```python
from build123d import *

# Parameters (mm, degrees)
EXTRUDE_1_DEPTH     = 3
SKETCH_5_R          = 1.65
CUT_EXTRUDE_1_DEPTH = 8


with BuildPart() as part:
    # Эскиз1 → Бобышка-Вытянуть1 (new body)
    with BuildSketch(Plane.XY):
        Polygon((0, 0), (0, 200), (50, 150), (50, 50), align=None)
    extrude(amount=EXTRUDE_1_DEPTH)

    # Эскиз5 → Вырез-Вытянуть1 (cut)
    with BuildSketch(Plane(origin=(-305.961161651, -184.204468703, -1.5), x_dir=(-0.9998892265297747, 0.01488404077153568, 0), z_dir=(0, 0, -1))):
        with BuildLine():
            ThreePointArc((-309.659295343, 358.877763083), (-310.142569154, 360.044489272), (-311.309295343, 360.527763083))
            Line((-311.309295343, 360.527763083), (-311.309295343, 357.227763083))
            ThreePointArc((-311.309295343, 357.227763083), (-310.142569154, 357.711036894), (-309.659295343, 358.877763083))
        make_face()
        with BuildLine():
            Line((-311.309295343, 357.227763083), (-311.309295343, 360.527763083))
            ThreePointArc((-311.309295343, 360.527763083), (-312.959295343, 358.877763083), (-311.309295343, 357.227763083))
        make_face()
        with Locations(Location((-311.309295343, 218.877763083, 0), (0, 0, 179.147175791))):
            Circle(SKETCH_5_R)
    extrude(amount=-CUT_EXTRUDE_1_DEPTH, mode=Mode.SUBTRACT)


solid = part.part
```
Here's how the part is built. I have some questions about the finished solid (model axes, mm). Coordinates: 2 decimals unless noted, no trailing zeros. Order: outer loops, then holes, each group sorted by start corner. A loop starts at its lowest first (then second) coordinate and runs counter-clockwise, first axis right, second up. Notation, with made-up numbers: M 59,78.5 L 97,78.5 A19 ccw 97,90.5 Z; hole C 17,77.25 d8. An arc over 180 degrees is marked long. Answer as a JSON object with one key per item and string values. Group by question number.
(1) Suppose I cut it at C-C, the plane x = 28. Please give me the cut outline in (y, z).
(2) I need wall thicknesses on probe 1 along Y at (x, z) = (10, 0.35); probe 2 along Y at (x, z) = (11.5, 2.75); probe 3 along X at (y, z) = (30, 1.05). Which ranges of each line are inside material? Lowest first, please.
(3) If we mould it in two halves opening along Y, with no side actions, what happens to faces 1 (the face through (25, 175, 1)), 2 (the face through (9.458, 28.624, 1.479)), 3 (the face through (20, 101, 3)), 4 (the face through (25, 25, 1))? For each: released by +Y, released by -Y, zero draft, split by the parting line, or undercut.
(4) For pin 1 (3 mm diameter, centred on x = 43, y = 39, fed in from +Z); pin 2 (1 mm diameter, centred on x = 12.5, y = 120, fed in from -Z); pin 3 (1 mm diameter, centred on x = 11, z = 2.5, fed in from +Y); pin 4 (1.5 mm diameter, centred on x = 18.5, z = 0.5, fed in from +Y), each with a flat end and sliding along its axis, tell me the tip position at first contact or that it passes through.
(5) Suppose I cut it at B-B, the plane y = 153. Please give me the cut outline in (x, z).
(6) Suppose I cut it at A-A, the plane z = 2.1. Please give me the cut outline in (x, y), then the cut area to 3 significant figures.
Values found:
{
 "1": {"outline": "M 28,0 L 172,0 L 172,3 L 28,3 Z"},
 "2": {"probe 1": "y = 10 to 29.19, 30.84 to 168.49, 171.51 to 190", "probe 2": "y = 11.5 to 168.58, 171.42 to 188.5", "probe 3": "x = 0 to 6.92, 10.22 to 30"},
 "3": {"face 1": "released by +Y", "face 2": "undercut", "face 3": "zero draft", "face 4": "released by -Y"},
 "4": {"pin 1": "passes through", "pin 2": "stops at z = 0", "pin 3": "stops at y = 189.5", "pin 4": "stops at y = 182.25"},
 "5": {"outline": "M 0,0 L 47,0 L 47,3 L 0,3 Z"},
 "6": {"outline": "M 0,0 L 50,50 L 50,150 L 0,200 Z; hole C 8.57,30.02 d3.3; hole C 10.66,170 d3.3", "area": "7,480 mm^2"}
}
